Source: CAD feature listing. Evaluate the final solid. Frame: model axes, mm. A direction names the side the tool comes from. Round coordinates to 2 decimals unless told otherwise and drop trailing zeros. Write each loop counter-clockwise with the first axis right and the second up, starting at its lowest first coordinate (ties: lowest second). Pieces come first, ordered by that corner, then holes. Notation, with made-up numbers: M 63.5,-10.5 L 70.5,-10.5 A16 cw 70.5,15.5 Z; hole C -3.5,-28.5 d10. An arc over 180 degrees is marked long. Answer in a Markdown table with one row per item. Add a question column.
Item 1: Contact query for flat-ended pins moving along their axis: pin 1 (3.5 mm diameter, centred on x = -100, z = -4, fed in from -Y); pin 2 (5 mm diameter, centred on x = -121, y = -18.5, fed in from -Z); pin 3 (7.5 mm diameter, centred on x = -91.5, y = 0.5, fed in from -Z); pin 4 (2.5 mm diameter, centred on x = 2.19, y = 20, fed in from +Z). Output: stop coordinate, or through.
Item 2: Cut plane A-A on y = 0. Return loops of the section in (x, z), and give its area (3 significant figures).
Item 3: Cut plane B-B on x = -13.81. Return loops of the section in (y, z).
Item 4: Mould query, pull axis X, two halves, no side actions, for faces 1 (the face through (-36.81, 0, -2)), 2 (the face through (-85, -10, -2)), 3 (the face through (1.93, 18.017, 2.81)), 4 (the face through (-34.855, 21.708, 7.88)). Classes: released by +X, released by -X, zero draft, split by the parting line, or undercut.
Item 5: Cut plane C-C on z = 3.75. Return loops of the section in (x, y), and give its area (3 significant figures).
Item 6: Cut plane D-D on x = -71. Return loops of the section in (y, z).
Item 7: Set-up query: faces 5 (the face through (-86, 7, -5)), 6 (the face through (-28.809, -18.217, 7.88)), 7 (the face through (-15, 25, 5)), 8 (the face through (-84, 3, -0.8)), 9 (the face through (-124.395, -0.047, 4.524)). Return all of +Z, -Z, +X, -X, +Y, -Y with unobstructed straight access to the full face (end or side cutting, diameter ignored); none if empty.
Item 8: Material intervals for probe 1 along Y at (x, z) = (2.19, 1.65); probe 2 along Y at (x, z) = (-13.81, 5); probe 3 along Y at (x, z) = (-49.5, -4), sorted ascending.
Autodesk Inventor part; units mm, degrees
ref_plane "YZ Plane" through (0, 0, 0) normal (1, 0, 0) x (0, 1, 0)
ref_plane "XZ Plane" through (0, 0, 0) normal (0, 1, 0) x (-1, 0, 0)
ref_plane "XY Plane" through (0, 0, 0) normal (0, 0, 1) x (1, 0, 0)
sketch "Skizze1" plane through (0, 0, 0) normal (0, 0, 1) x (1, 0, 0)
  circle A0 centre (2.19, 20) radius 2
  circle A1 centre (-31.81, 20) radius 2
  arc A2 (-31.81, 25) -> (-36.81, 20) centre (-31.81, 20) ccw
  line L0 (-36.81, 20) -> (-36.81, 16)
  line L1 (7.19, 16) -> (7.19, 20)
  arc A3 (7.19, 20) -> (2.19, 25) centre (2.19, 20) ccw
  line L2 (2.19, 25) -> (-31.81, 25)
  circle A4 centre (2.19, -20) radius 2
  circle A5 centre (-31.81, -20) radius 2
  arc A6 (-36.81, -20) -> (-31.81, -25) centre (-31.81, -20) ccw
  line L3 (-31.81, -25) -> (2.19, -25)
  arc A7 (2.19, -25) -> (7.19, -20) centre (2.19, -20) ccw
  line L4 (7.19, -20) -> (7.19, -16)
  line L5 (-36.81, -16) -> (-36.81, -20)
  line L6 (-29.81, -10) -> (-36.81, -10)
  line L7 (-36.81, -16) -> (-36.81, -10)
  line L8 (7.19, 16) -> (7.19, -16)
  line L9 (-36.81, 10) -> (-36.81, 16)
  line L10 (-36.81, 10) -> (-29.81, 10)
  line L11 (-29.81, 10) -> (-29.81, -10)
  circle A8 centre (-13.81, 0) radius 8
  point P0 (0, 0)
extrude "Extrusion1" add sketch "Skizze1" along normal blind 10
sketch "Skizze3" plane through (-36.81, 10, 0) normal (-1, 0, 0) x (0, 0, 1)
  line L0 (0, 10) -> (0, 0)
  line L1 (0, 0) -> (10, 0)
  line L2 (10, 10) -> (10, 0)
  line L3 (0, 10) -> (10, 10)
  line L4 (0, -20) -> (0, -30)
  line L5 (0, -30) -> (10, -30)
  line L6 (10, -20) -> (10, -30)
  line L7 (0, -20) -> (10, -20)
  line L8 (10, -0.1675) -> (10, -20.1669)
  line L9 (0, 0) -> (0, -20)
  line L10 (10, -35) -> (10, -30)
  line L11 (0, 10) -> (10, 10)
  line L12 (10, 10) -> (10, -30)
  line L13 (10, -30) -> (0, -30)
  line L14 (0, -30) -> (0, 10)
  point P0 (0, -10)
extrude "Extrusion3" add sketch "Skizze3" along normal blind 100
sketch "Skizze4" plane through (0, 0, 10) normal (0, 0, 1) x (1, 0, 0)
  line L0 (-36.81, 20) -> (-136.81, 20)
  arc A0 (-31.81, 25) -> (-36.81, 20) centre (-31.81, 20) ccw
  line L1 (-36.81, 20) -> (-136.81, 20)
  arc A1 (-31.81, 25) -> (-36.81, 20) centre (-31.81, 20) ccw
  arc A2 (-45.8607, 20) -> (-35.3455, 23.5355) centre (-45.0384, 34.959) ccw
  line L2 (-44.2162, 20) -> (-36.81, 20)
  arc A3 (-35.3455, 23.5355) -> (-36.81, 20) centre (-31.81, 20) ccw
  line L3 (-45.8607, 0) -> (-28.5304, 0)
  line L4 (-36.81, -20) -> (-136.81, -20)
  arc A4 (-36.81, -20) -> (-31.81, -25) centre (-31.81, -20) ccw
  arc A5 (-35.3455, -23.5355) -> (-45.8607, -20) centre (-45.0384, -34.959) ccw
  line L5 (-36.81, -20) -> (-136.81, -20)
  line L6 (-44.2159, -20) -> (-36.81, -20)
  arc A6 (-36.81, -20) -> (-31.81, -25) centre (-31.81, -20) ccw
  arc A7 (-36.81, -20) -> (-31.81, -25) centre (-31.81, -20) ccw
  arc A8 (-35.1548, -23.7165) -> (-45.8607, -20) centre (-44.9788, -34.7378) ccw
  point P0 (0, 0)
extrude "Extrusion4" add sketch "Skizze4" against normal blind 10 contours L0 A2 A0 | L4 A4 A5 A8
fillet "Rundung1" radius 5 2 edges at (-136.81, 20, 5) (-136.81, -20, 5)
sketch "Skizze10" plane through (0, 0, 0) normal (0, 0, -1) x (-1, 0, 0)
  line L0 (36.8821, 9.8325) -> (29.8823, 9.8834) construction
  line L1 (29.7369, -10.116) -> (36.7367, -10.1669) construction
  line L2 (36.81, 10) -> (29.81, 10)
  line L3 (29.81, -10) -> (36.81, -10)
  line L4 (136.81, 15) -> (136.81, -15)
  line L5 (36.81, 10) -> (136.81, 10)
  line L6 (136.81, 10) -> (136.81, -10)
  line L7 (136.81, -10) -> (36.81, -10)
  line L8 (36.81, -10) -> (36.81, 10)
  point P0 (0, 0)
extrude "Extrusion10" add sketch "Skizze10" along normal blind 5
fillet "Rundung3" radius 5 2 edges at (-136.81, 10, -2.5) (-136.81, -10, -2.5)
sketch "Skizze11" plane through (0, 0, -5) normal (0, 0, -1) x (-1, 0, 0)
  line L0 (131.81, 10) -> (36.81, 10) construction
  line L1 (36.81, -10) -> (131.81, -10) construction
  line L2 (40.8, 0) -> (128.9956, 0) construction
  line L3 (45.4, -4.6) -> (124.3956, -4.6)
  line L4 (124.3956, 4.6) -> (45.4, 4.6)
  arc A0 (45.4, 4.6) -> (45.4, -4.6) centre (45.4, 0) ccw
  arc A1 (124.3956, -4.6) -> (124.3956, 4.6) centre (124.3956, 0) ccw
  point P0 (0, 0)
  point P1 (84.8978, 0)
  dimension "d40" = 9.2
extrude "Extrusion11" cut sketch "Skizze11" against normal blind 4.2
sketch "Skizze12" plane through (0, 0, -0.8) normal (0, 0, -1) x (-1, 0, 0)
  line L0 (124.3956, -4.6) -> (45.4, -4.6)
  arc A0 (124.3956, -4.6) -> (124.3956, 4.6) centre (124.3956, 0) ccw
  line L1 (45.4, 4.6) -> (124.3956, 4.6)
  arc A1 (45.4, 4.6) -> (45.4, -4.6) centre (45.4, 0) ccw
  line L2 (45.4, 0) -> (124.3956, 0) construction
  line L3 (47.55, -2.15) -> (122.2456, -2.15)
  line L4 (122.2456, 2.15) -> (47.55, 2.15)
  arc A2 (47.55, 2.15) -> (47.55, -2.15) centre (47.55, 0) ccw
  arc A3 (122.2456, -2.15) -> (122.2456, 2.15) centre (122.2456, 0) ccw
  point P0 (0, 0)
  point P1 (84.8978, 0)
  dimension "d43" = 4.3
extrude "Extrusion12" cut sketch "Skizze12" against normal through all contours A2 L4 A3 L3
sketch "Skizze13" plane through (0, 0, 10) normal (0, 0, 1) x (1, 0, 0)
  circle A0 centre (-31.81, 20) radius 2 construction
  circle A1 centre (2.19, 20) radius 2 construction
  circle A2 centre (2.19, -20) radius 2 construction
  circle A3 centre (-31.81, -20) radius 2 construction
  line L0 (-31.81, 20) -> (2.19, 20) construction
  line L1 (2.19, 20) -> (2.19, -20) construction
  line L2 (-31.81, 20) -> (-31.81, 23.5) construction
  line L3 (-31.81, 23.5) -> (-29.9614, 23.5)
  line L4 (-29.9614, 23.5) -> (-33.1306, 23.5)
  line L5 (-29.81, 23.5) -> (-27.7789, 20.0179)
  line L6 (-27.7789, 20.0179) -> (-29.7789, 16.5179)
  line L7 (-29.7789, 16.5179) -> (-33.81, 16.5)
  line L8 (-33.81, 16.5) -> (-35.8411, 19.9821)
  line L9 (-35.8411, 19.9821) -> (-33.8411, 23.4821)
  line L10 (-33.8411, 23.4821) -> (-29.81, 23.5)
  line L11 (2.19, 20) -> (2.19, 23.5) construction
  line L12 (2.19, 23.5) -> (4.0386, 23.5)
  line L13 (4.0386, 23.5) -> (0.8694, 23.5)
  line L14 (4.19, 23.5) -> (6.2211, 20.0179)
  line L15 (6.2211, 20.0179) -> (4.2211, 16.5179)
  line L16 (4.2211, 16.5179) -> (0.19, 16.5)
  line L17 (0.19, 16.5) -> (-1.8411, 19.9821)
  line L18 (-1.8411, 19.9821) -> (0.1589, 23.4821)
  line L19 (0.1589, 23.4821) -> (4.19, 23.5)
  line L20 (-31.81, -20) -> (-31.81, -16.5) construction
  line L21 (-31.81, -16.5) -> (-29.9614, -16.5)
  line L22 (-29.9614, -16.5) -> (-33.1306, -16.5)
  line L23 (-29.81, -16.5) -> (-27.7789, -19.9821)
  line L24 (-27.7789, -19.9821) -> (-29.7789, -23.4821)
  line L25 (-29.7789, -23.4821) -> (-33.81, -23.5)
  line L26 (-33.81, -23.5) -> (-35.8411, -20.0179)
  line L27 (-35.8411, -20.0179) -> (-33.8411, -16.5179)
  line L28 (-33.8411, -16.5179) -> (-29.81, -16.5)
  line L29 (2.19, -20) -> (2.19, -16.5) construction
  line L30 (2.19, -16.5) -> (4.0386, -16.5)
  line L31 (4.0386, -16.5) -> (0.8694, -16.5)
  line L32 (4.19, -16.5) -> (6.2211, -19.9821)
  line L33 (6.2211, -19.9821) -> (4.2211, -23.4821)
  line L34 (4.2211, -23.4821) -> (0.19, -23.5)
  line L35 (0.19, -23.5) -> (-1.8411, -20.0179)
  line L36 (-1.8411, -20.0179) -> (0.1589, -16.5179)
  line L37 (0.1589, -16.5179) -> (4.19, -16.5)
  point P0 (0, 0)
  dimension "d61" = 3.5
  dimension "d64" = 34
  dimension "d67" = 40
extrude "Extrusion14" cut sketch "Skizze13" against normal blind 4.3
sketch "Skizze14" plane through (0, 0, 0) normal (0, 0, -1) x (-1, 0, 0)
  line L0 (29.81, 10) -> (29.81, -10)
  line L1 (36.81, 10) -> (29.81, 10)
  line L2 (36.81, -16.5129) -> (36.81, 16.5129)
  line L3 (29.81, -10) -> (36.81, -10)
  point P0 (0, 0)
extrude "Extrusion15" add sketch "Skizze14" against normal up to surface (10 mm away)
properties part number "Bearing_support_inside"
Results below:
| question | item | result |
|---|---|---|
| 1 | pin 1 | y = -10 |
| 1 | pin 2 | z = 0 |
| 1 | pin 3 | z = -0.8 |
| 1 | pin 4 | through |
| 2 | outline | M -136.81,-5 L -129,-5 L -129,-0.8 L -124.4,-0.8 L -124.4,10 L -136.81,10 Z; M -45.4,-0.8 L -40.8,-0.8 L -40.8,-5 L -36.81,-5 L -36.81,0 L -21.81,0 L -21.81,10 L -45.4,10 Z; M -5.81,0 L 7.19,0 L 7.19,10 L -5.81,10 Z |
| 2 | area | 556 mm2 |
| 3 | outline | M -25,0 L -8,0 L -8,10 L -25,10 Z; M 8,0 L 25,0 L 25,10 L 8,10 Z |
| 4 | face 1 | released by +X |
| 4 | face 2 | zero draft |
| 4 | face 3 | undercut |
| 4 | face 4 | undercut |
| 5 | outline | M -136.81,-15 A5 ccw -131.81,-20 L -44.1,-20 A14.76 cw -36.82,-22.43 A14.98 cw -35.35,-23.54 A5 ccw -31.81,-25 L 2.19,-25 A5 ccw 7.19,-20 L 7.19,20 A5 ccw 2.19,25 L -31.81,25 A5 ccw -35.35,23.54 A14.98 cw -44.22,20 L -131.81,20 A5 ccw -136.81,15 Z; hole M -122.25,-2.15 L -47.55,-2.15 A2.15 ccw -47.55,2.15 L -122.25,2.15 A2.15 ccw Z; hole C -31.81,-20 d4; hole C -31.81,20 d4; hole C -13.81,0 d16; hole C 2.19,-20 d4; hole C 2.19,20 d4 |
| 5 | area | 5,590 mm2 |
| 6 | outline | M -20,0 L -10,0 L -10,-5 L -4.6,-5 L -4.6,-0.8 L -2.15,-0.8 L -2.15,10 L -20,10 Z; M 2.15,-0.8 L 4.6,-0.8 L 4.6,-5 L 10,-5 L 10,0 L 20,0 L 20,10 L 2.15,10 Z |
| 7 | face 5 | -Z, +X, -X, +Y, -Y |
| 7 | face 6 | +Z |
| 7 | face 7 | +Z, -Z, +X, -X, +Y |
| 7 | face 8 | -Z |
| 7 | face 9 | +Z, -Z |
| 8 | probe 1 | -25 to -22, -18 to 18, 22 to 25 |
| 8 | probe 2 | -25 to -8, 8 to 25 |
| 8 | probe 3 | -10 to -4.6, 4.6 to 10 |
